from build123d import *

# Parameters (mm, degrees)
SKETCH_1_R      = 1.6
SKETCH_1_R_2    = 1.1
EXTRUDE_1_DEPTH = 3
FILLET_2_R      = 4


with BuildPart() as part:
    # 草图1 → 凸台-拉伸1 (new body)
    with BuildSketch(Plane.XY):
        with BuildLine():
            Line((-31, 25.46), (31, 25.46))
            Line((31, 25.46), (31, -25.46))
            Line((31, -25.46), (-31, -25.46))
            ThreePointArc((-31, -25.46), (-35.614835193, -22.497087982), (-41, -21.46))
            Line((-41, -21.46), (-56.07, -21.46))
            ThreePointArc((-56.07, -21.46), (-61.07, -16.46), (-56.07, -11.46))
            Line((-56.07, -11.46), (-41, -11.46))
            ThreePointArc((-41, -11.46), (-33.928932188, -8.531067812), (-31, -1.46))
            Line((-31, -1.46), (-31, 25.46))
        make_face()
        with Locations((-27, 21.46)):
            Circle(SKETCH_1_R, mode=Mode.SUBTRACT)
        with Locations((27, 21.46)):
            Circle(SKETCH_1_R, mode=Mode.SUBTRACT)
        with Locations((-27, -21.46)):
            Circle(SKETCH_1_R, mode=Mode.SUBTRACT)
        with Locations((27, -21.46)):
            Circle(SKETCH_1_R, mode=Mode.SUBTRACT)
        with Locations((-11.5, 16.5)):
            Circle(SKETCH_1_R_2, mode=Mode.SUBTRACT)
        with Locations((11.5, 16.5)):
            Circle(SKETCH_1_R_2, mode=Mode.SUBTRACT)
        with Locations((11.5, -16.5)):
            Circle(SKETCH_1_R_2, mode=Mode.SUBTRACT)
        with Locations((-11.5, -16.5)):
            Circle(SKETCH_1_R_2, mode=Mode.SUBTRACT)
        with Locations((-56.07, -16.46)):
            Circle(SKETCH_1_R_2, mode=Mode.SUBTRACT)
        with Locations((-37, -16.46)):
            Circle(SKETCH_1_R_2, mode=Mode.SUBTRACT)
        with BuildLine():
            Line((-22.510011136, 20.46), (-18.534799215, 20.46))
            ThreePointArc((-18.534799215, 20.46), (-16.274611014, 19.432701015), (-15.562348843, 17.054366197))
            ThreePointArc((-15.562348843, 17.054366197), (-11.5, 12.4), (-7.437651157, 17.054366197))
            ThreePointArc((-7.437651157, 17.054366197), (-6.725388986, 19.432701015), (-4.465200785, 20.46))
            Line((-4.465200785, 20.46), (4.465200785, 20.46))
            ThreePointArc((4.465200785, 20.46), (6.725388986, 19.432701015), (7.437651157, 17.054366197))
            ThreePointArc((7.437651157, 17.054366197), (11.5, 12.4), (15.562348843, 17.054366197))
            ThreePointArc((15.562348843, 17.054366197), (16.274611014, 19.432701015), (18.534799215, 20.46))
            Line((18.534799215, 20.46), (22.510011136, 20.46))
            ThreePointArc((22.510011136, 20.46), (23.747308807, 18.207308807), (26, 16.970011136))
            Line((26, 16.970011136), (26, -16.970011136))
            ThreePointArc((26, -16.970011136), (23.747308807, -18.207308807), (22.510011136, -20.46))
            Line((22.510011136, -20.46), (18.534799215, -20.46))
            ThreePointArc((18.534799215, -20.46), (16.274611014, -19.432701015), (15.562348843, -17.054366197))
            ThreePointArc((15.562348843, -17.054366197), (11.5, -12.4), (7.437651157, -17.054366197))
            ThreePointArc((7.437651157, -17.054366197), (6.725388986, -19.432701015), (4.465200785, -20.46))
            Line((4.465200785, -20.46), (-4.465200785, -20.46))
            ThreePointArc((-4.465200785, -20.46), (-6.725388986, -19.432701015), (-7.437651157, -17.054366197))
            ThreePointArc((-7.437651157, -17.054366197), (-11.5, -12.4), (-15.562348843, -17.054366197))
            ThreePointArc((-15.562348843, -17.054366197), (-16.274611014, -19.432701015), (-18.534799215, -20.46))
            Line((-18.534799215, -20.46), (-21.4, -20.46))
            ThreePointArc((-21.4, -20.46), (-24.652691193, -19.112691193), (-26, -15.86))
            Line((-26, -15.86), (-26, 16.970011136))
            ThreePointArc((-26, 16.970011136), (-23.747308807, 18.207308807), (-22.510011136, 20.46))
        make_face(mode=Mode.SUBTRACT)
    extrude(amount=EXTRUDE_1_DEPTH)

    # 圆角2
    fillet_2_edges = [part.edges().sort_by_distance(p)[0] for p in [
        (-31, 25.46, 1.5),
        (31, 25.46, 1.5),
        (31, -25.46, 1.5),
    ]]
    fillet(fillet_2_edges, radius=FILLET_2_R)


solid = part.part
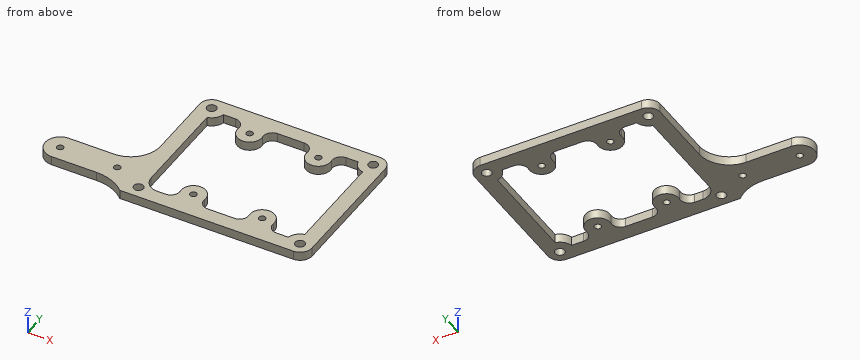
The model under review builds one solid part; all positions refer to its coordinate system, in mm. Coordinates: 2 decimals unless noted, no trailing zeros. Loops run counter-clockwise (first coordinate to the right, second up) from the corner with the lowest first, then second, coordinate; pieces in that order, holes last. Notation, with made-up numbers: (88.25, 85.25) -> (95.25, 85.25) arc R35 cw to (95.25, 120.25) -> close; hole circle Ø1 at (-25.5, -30.75). An arc over 180 degrees is marked (long way). Use a Markdown table: item, result. Add a question column.
1. Add section A-A on y = 1. Write out the cut boundary in (x, z), plus the area to 3 significant figures.
2. Add section C-C on x = -53.5. Write out the cut boundary in (y, z).
3. Add section B-B on x = -11.5. Write out the cut boundary in (y, z), plus the area to 3 significant figures.
4. Add section D-D on z = 1.5. Give the number of separate pieces and of enclosed holes in the cut face, plus the area to 3 significant figures.
5. Clearance check with flat-ended pins moving along their axes: pin 1 Ø0.9 at (y, z) = (6, 1.5) entering from -X; pin 2 Ø3.5 at (x, y) = (-11.5, 16.5) entering from -Z; pin 3 Ø0.9 at (x, z) = (-47.5, 1.5) entering from -Y. State where each tip first meets the part, or that it passes through.
6. To check wall thickness, follow line 1 (X direction, y = 11, z = 0.85); line 2 (X direction, y = -21, z = 0.95); line 3 (X direction, y = -19.5, z = 1.05). State the ranges of each line that lie inside material, in increasing order.
Returned:
| question | item | result |
|---|---|---|
| 1 | outline | (-31, 0) -> (-26, 0) -> (-26, 3) -> (-31, 3) -> close; (26, 0) -> (31, 0) -> (31, 3) -> (26, 3) -> close |
| 1 | area | 30.0 mm² |
| 2 | outline | (-21.46, 0) -> (-11.46, 0) -> (-11.46, 3) -> (-21.46, 3) -> close |
| 3 | outline | (-25.46, 0) -> (-17.6, 0) -> (-17.6, 3) -> (-25.46, 3) -> close; (-15.4, 0) -> (-12.4, 0) -> (-12.4, 3) -> (-15.4, 3) -> close; (12.4, 0) -> (15.4, 0) -> (15.4, 3) -> (12.4, 3) -> close; (17.6, 0) -> (25.46, 0) -> (25.46, 3) -> (17.6, 3) -> close |
| 3 | area | 65.2 mm² |
| 4 | separate pieces | 1 |
| 4 | enclosed holes | 11 |
| 4 | area | 1,570 mm² |
| 5 | pin 1 | stops at x = -31 |
| 5 | pin 2 | stops at z = 0 |
| 5 | pin 3 | stops at y = -21.46 |
| 6 | line 1 | x = -31 to -26, 26 to 31 |
| 6 | line 2 | x = -58.16 to -28.53, -25.47 to 25.47, 28.53 to 31 |
| 6 | line 3 | x = -60.04 to -24.21, -16.34 to -6.66, 6.66 to 16.34, 22.84 to 31 |
